```python
from build123d import *

# Parameters (mm, degrees)
SKETCH_3_W          = 60
SKETCH_3_H          = 60
SKETCH_3_R          = 10
EXTRUDE_2_DEPTH     = 5
SKETCH_4_R          = 2.1
CUT_EXTRUDE_1_DEPTH = 5


with BuildPart() as part:
    # 草图3 → 凸台-拉伸2 (new body)
    with BuildSketch(Plane.XY):
        Rectangle(SKETCH_3_W, SKETCH_3_H)
        Circle(SKETCH_3_R, mode=Mode.SUBTRACT)
    extrude(amount=EXTRUDE_2_DEPTH)

    # 草图4 → 切除-拉伸1 (cut)
    with BuildSketch(Plane.XY):
        with Locations(Location((11.875, 20.56810334, 0), (0, 0, 180))):
            Circle(SKETCH_4_R)
        with Locations(Location((22.5, 0, 0), (0, 0, 180))):
            Circle(SKETCH_4_R)
        with Locations(Location((11.875, -20.56810334, 0), (0, 0, 180))):
            Circle(SKETCH_4_R)
        with Locations(Location((-11.25, -19.485571585, 0), (0, 0, 180))):
            Circle(SKETCH_4_R)
        with Locations(Location((-23.75, 0, 0), (0, 0, 180))):
            Circle(SKETCH_4_R)
        with Locations(Location((-11.25, 19.485571585, 0), (0, 0, 180))):
            Circle(SKETCH_4_R)
        with Locations(Location((-23.75, 23.75, 0), (0, 0, 180))):
            Circle(SKETCH_4_R)
        with Locations(Location((23.75, 23.75, 0), (0, 0, 180))):
            Circle(SKETCH_4_R)
        with Locations(Location((23.75, -23.75, 0), (0, 0, 180))):
            Circle(SKETCH_4_R)
        with Locations(Location((-23.75, -23.75, 0), (0, 0, 180))):
            Circle(SKETCH_4_R)
    extrude(amount=CUT_EXTRUDE_1_DEPTH, mode=Mode.SUBTRACT)


solid = part.part
```
Read the model definition and answer for the solid it produces. Units are mm, in the model's axes. Give positions to 0.01 mm unless a question says otherwise; leave off trailing zeros. Order: outer loops, then holes, each group sorted by start corner. A loop starts at its lowest first (then second) coordinate and runs counter-clockwise, first axis right, second up. Notation, with made-up numbers: (23.5, 7) -> (77.5, 7) arc R32 ccw to (77.5, 36) -> close; hole circle Ø2 at (62.5, -25.75). An arc over 180 degrees is marked (long way). One line per item, written item: value. Start each with the question number.
(1) The part is cut by section B-B (y = -23.75). Determine the outline of the cut face in (x, z), and give its area (3 significant figures).
(2) Flat-ended cylindrical pins translate along their axes: P1, Ø6.5, axis at x = 11.88, y = 20.57, coming from the -Z side; P2, Ø4, axis at x = 23.75, y = -23.75, coming from the -Z side. Find the tip coordinate at first contact, or state that the pin passes through.
(3) For a pull along X with two mould halves and no side action, classify faces 1 (the cylindrical face through (-9.152, 19.393, 2.465)), 2 (the flat face through (30, 0, 2)), 3 (the flat face through (0, -30, 2)) as released by +X, released by -X, zero draft, split by the parting line, or undercut.
(4) Straight lines are drawn through the part: L1, parallel to Y at x = -11.25, z = 2.2; L2, parallel to Y at x = -23.75, z = 1.15; L3, parallel to Y at x = 23.75, z = 3.8. For each, find the intervals that lie inside material, in ascending order.
(5) The part is cut by section C-C (x = -23.75). Determine the outline of the cut face in (y, z).
(6) The part is cut by section A-A (x = -11.25). Determine the outline of the cut face in (y, z), and give its area (3 significant figures).
(7) The part is cut by section D-D (x = 0). Determine the outline of the cut face in (y, z), and give its area (3 significant figures).
Taken from the geometry:
1. outline: (-30, 0) -> (-25.85, 0) -> (-25.85, 5) -> (-30, 5) -> close; (-21.65, 0) -> (21.65, 0) -> (21.65, 5) -> (-21.65, 5) -> close; (25.85, 0) -> (30, 0) -> (30, 5) -> (25.85, 5) -> close
1. area: 258 mm^2
2. P1: z = 0
2. P2: through
3. face 1: undercut
3. face 2: released by +X
3. face 3: zero draft
4. L1: -30 to -21.59, -17.39 to 17.39, 21.59 to 30
4. L2: -30 to -25.85, -21.65 to -2.1, 2.1 to 21.65, 25.85 to 30
4. L3: -30 to -25.85, -21.65 to -1.69, 1.69 to 21.65, 25.85 to 30
5. outline: (-30, 0) -> (-25.85, 0) -> (-25.85, 5) -> (-30, 5) -> close; (-21.65, 0) -> (-2.1, 0) -> (-2.1, 5) -> (-21.65, 5) -> close; (2.1, 0) -> (21.65, 0) -> (21.65, 5) -> (2.1, 5) -> close; (25.85, 0) -> (30, 0) -> (30, 5) -> (25.85, 5) -> close
6. outline: (-30, 0) -> (-21.59, 0) -> (-21.59, 5) -> (-30, 5) -> close; (-17.39, 0) -> (17.39, 0) -> (17.39, 5) -> (-17.39, 5) -> close; (21.59, 0) -> (30, 0) -> (30, 5) -> (21.59, 5) -> close
6. area: 258 mm^2
7. outline: (-30, 0) -> (-10, 0) -> (-10, 5) -> (-30, 5) -> close; (10, 0) -> (30, 0) -> (30, 5) -> (10, 5) -> close
7. area: 200 mm^2
